```python
from build123d import *

# Parameters (mm, degrees)
F0_W     = 50
F0_H     = 50
F1_DEPTH = 5
F2_R     = 5
F3_DEPTH = 25
F5_DEPTH = 25


with BuildPart() as f1:
    # F0 (on Top) → F1 (new body)
    with BuildSketch(Plane.XY):
        Rectangle(F0_W, F0_H)
    extrude(amount=F1_DEPTH)

    # F2 (on face) → F3 (cut)
    with BuildSketch(Plane.XY.offset(5)):
        Circle(F2_R)
    extrude(amount=-F3_DEPTH, mode=Mode.SUBTRACT)

    # F4 (on face) → F5 (cut)
    with BuildSketch(Plane.XY.offset(5)):
        with BuildLine():
            add(Edge.make_bspline(
                [(-16.0939358175, 19.4073952734), (-12.4173646388, 20.576681651), (-2.1134920052, 20.3363583902), (-5.8241318664, 9.2256089441), (-17.5792885427, 4.957394915), (-22.4856509352, 14.9328212493), (-18.9737953325, 18.491492837), (-16.0939358175, 19.4073952734)],
                knots=[0, 0, 0, 0, 0.2259129236, 0.4146370942, 0.6325225982, 0.8230423264, 1, 1, 1, 1], degree=3))
        make_face()
    extrude(amount=-F5_DEPTH, mode=Mode.SUBTRACT)


solid = f1.part
```
Model file for the job. Use its own axes, mm. Coordinates: 2 decimals unless noted, no trailing zeros. Loops run counter-clockwise (first coordinate to the right, second up) from the corner with the lowest first, then second, coordinate; pieces in that order, holes last. Notation, with made-up numbers: M -4.5,35.25 L 49.5,35.25 A28 cw 49.5,71.25 Z; hole C 58.25,19 d8. An arc over 180 degrees is marked long. Use CSV: the item, a comma, the result in double quotes. Start each with the question number.
1. Band-saw the part on A-A, the plane x = 0. List the corners of the cut face in (y, z), then the cut area to 3 significant figures.
2. Probe probe 1 along Y at (x, z) = (0, 2.25); probe 2 along X at (y, z) = (-1, 1.7); probe 3 along X at (y, z) = (8.5, 4.15). List the from-to ranges inside material, lowest first. Write a range as [from, to].
3. Band-saw the part on C-C, the plane z = 1.9. Give the number of separate pieces and of enclosed holes in the cut face, then the cut area to 3 significant figures.
4. Two-plate mould, pull along X, no slides. Class faces 1 (the flat face through (25, 0, 2)), 2 (the flat face through (0, 25, 2)), 3 (the flat face through (-25, 0, 2)), 4 (the cylindrical face through (-1.08, -4.88, 2.54)): pulls with the +X half, pulls with the -X half, needs draft (parallel to the pull), parting line crosses it, or undercut.
Entries:
1,outline,"M -25,0 L -5,0 L -5,5 L -25,5 Z; M 5,0 L 25,0 L 25,5 L 5,5 Z"
1,area,"200 mm2"
2,probe 1,"y = [-25, -5], [5, 25]"
2,probe 2,"x = [-25, -4.9], [4.9, 25]"
2,probe 3,"x = [-25, -18.28], [-9.67, 25]"
3,separate pieces,"1"
3,enclosed holes,"2"
3,area,"2,250 mm2"
4,face 1,"pulls with the +X half"
4,face 2,"needs draft"
4,face 3,"pulls with the -X half"
4,face 4,"undercut"
